Answer from the drawing. Dimensions are ordinates in mm from the lowest x, y and z of the part. Round coordinates to 2 decimals unless told otherwise and drop trailing zeros. Loops run counter-clockwise (first coordinate to the right, second up) from the corner with the lowest first, then second, coordinate; pieces in that order, holes last. Notation, with made-up numbers: (87.5, -1.5) -> (134.5, -1.5) arc R16 ccw to (134.5, 2.5) -> close; hole circle Ø3 at (48, -10). An arc over 180 degrees is marked (long way). One line per question, with ' | ' between items.
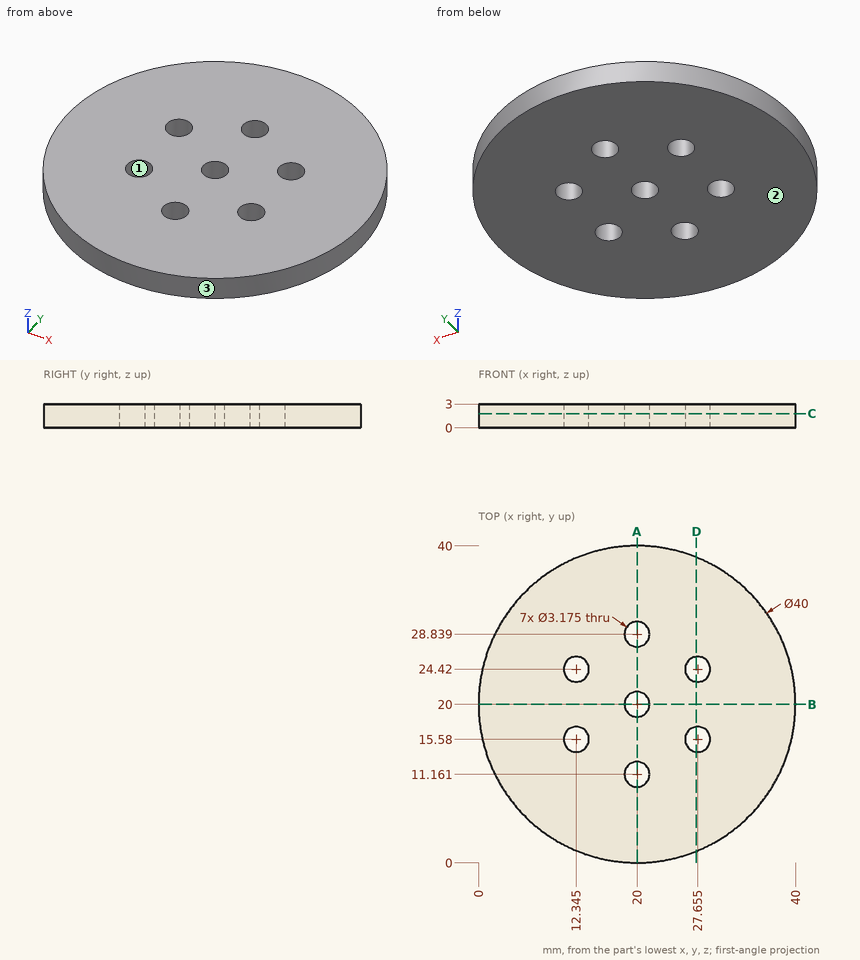
Q1. Given pin 1 Ø1.9 at (x, y) = (12.34, 15.58) entering from -Z; pin 2 Ø1.5 at (y, z) = (6.5, 2) entering from +X; pin 3 Ø1 at (x, z) = (4.5, 2) entering from -Y, each flat-ended and moving along its own axis, determine where each tip first touches the part or whether it passes through.
Numbers:
pin 1: through | pin 2: x = 35.41 | pin 3: y = 6.77
Q2. A cutting plane is placed at B-B on y = 20. Give the vertices of the cut face in (x, z).
Numbers:
outline: (0, 0) -> (18.41, 0) -> (18.41, 3) -> (0, 3) -> close; (21.59, 0) -> (40, 0) -> (40, 3) -> (21.59, 3) -> close
Q3. A cutting plane is placed at C-C on z = 1.8. Give the vertices of the cut face in (x, y) (1 decimal), plus the area to 3 significant figures.
Numbers:
outline: circle Ø40 at (20, 20); hole circle Ø3.2 at (12.3, 15.6); hole circle Ø3.2 at (12.3, 24.4); hole circle Ø3.2 at (20, 11.2); hole circle Ø3.2 at (20, 20); hole circle Ø3.2 at (20, 28.8); hole circle Ø3.2 at (27.7, 15.6); hole circle Ø3.2 at (27.7, 24.4) | area: 1,200 mm^2
Q4. A cutting plane is placed at D-D on x = 27.5. Give the vertices of the cut face in (y, z).
Numbers:
outline: (1.46, 0) -> (14, 0) -> (14, 3) -> (1.46, 3) -> close; (17.16, 0) -> (22.84, 0) -> (22.84, 3) -> (17.16, 3) -> close; (26, 0) -> (38.54, 0) -> (38.54, 3) -> (26, 3) -> close
Q5. Find the intervals of material crossed by line 1 (Y direction, x = 20, z = 0.9); line 2 (Y direction, x = 29, z = 1.7) (1 decimal); line 3 (Y direction, x = 28.5, z = 0.3) (1 decimal), in increasing order. Write a range as from..to.
Numbers:
line 1: 0..9.57, 12.75..18.41, 21.59..27.25, 30.43..40 | line 2: 2.1..14.7, 16.4..23.6, 25.3..37.9 | line 3: 1.9..14.2, 16.9..23.1, 25.8..38.1
Q6. A cutting plane is placed at A-A on x = 20. Give the vertices of the cut face in (y, z).
Numbers:
outline: (0, 0) -> (9.57, 0) -> (9.57, 3) -> (0, 3) -> close; (12.75, 0) -> (18.41, 0) -> (18.41, 3) -> (12.75, 3) -> close; (21.59, 0) -> (27.25, 0) -> (27.25, 3) -> (21.59, 3) -> close; (30.43, 0) -> (40, 0) -> (40, 3) -> (30.43, 3) -> close
Q7. For a pull along X with two mould halves and no side action, classify the marked faces 1, 2 and 3 as pulls with the +X half, pulls with the -X half, needs draft (parallel to the pull), parting line crosses it, or undercut.
Numbers:
face 1: undercut | face 2: needs draft | face 3: parting line crosses it
